```python
from build123d import *

# Parameters (mm, degrees)
SKETCH1_W           = 235
SKETCH1_H           = 120
BOSS_EXTRUDE1_DEPTH = 10
SKETCH2_R           = 15
CUT_EXTRUDE1_DEPTH  = 10
SKETCH3_R           = 2.5
CUT_EXTRUDE2_DEPTH  = 10


with BuildPart() as part:
    # Sketch1 → Boss-Extrude1 (new body)
    with BuildSketch(Plane.XY):
        Rectangle(SKETCH1_W, SKETCH1_H)
    extrude(amount=BOSS_EXTRUDE1_DEPTH)

    # Sketch2 → Cut-Extrude1 (cut)
    with BuildSketch(Plane.XY.offset(10)):
        Circle(SKETCH2_R)
    extrude(amount=-CUT_EXTRUDE1_DEPTH, mode=Mode.SUBTRACT)

    # Sketch3 → Cut-Extrude2 (cut)
    with BuildSketch(Plane.XY.offset(10)):
        with Locations((31.819805153, 31.819805153)):
            Circle(SKETCH3_R)
        with Locations((31.819805153, -31.819805153)):
            Circle(SKETCH3_R)
        with Locations((-31.819805153, -31.819805153)):
            Circle(SKETCH3_R)
        with Locations((-31.819805153, 31.819805153)):
            Circle(SKETCH3_R)
    extrude(amount=-CUT_EXTRUDE2_DEPTH, mode=Mode.SUBTRACT)


solid = part.part
```
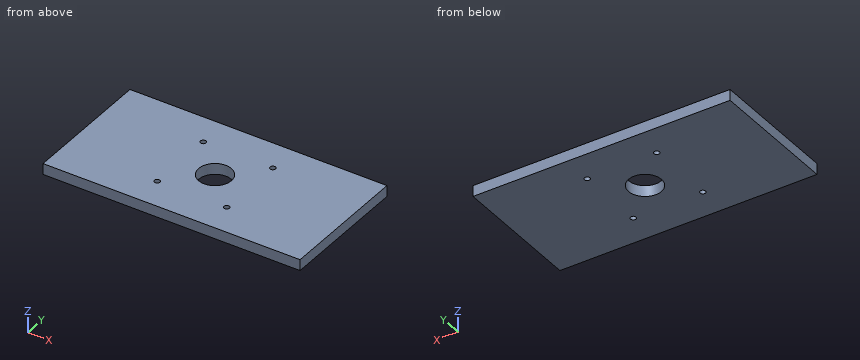
Input: part model. Units: mm. Frame: model coordinates. Give positions to 0.01 mm unless a question says otherwise; leave off trailing zeros. Loops run counter-clockwise (first coordinate to the right, second up) from the corner with the lowest first, then second, coordinate; pieces in that order, holes last.
1) Line query: L1, parallel to X at y = 0.5, z = 7.25; L2, parallel to X at y = -30, z = 0.5; L3, parallel to X at y = -2.5, z = 0.5. Output: solid intervals per line, ascending.
A:
L1: x = -117.5 to -14.99, 14.99 to 117.5
L2: x = -117.5 to -33.53, -30.11 to 30.11, 33.53 to 117.5
L3: x = -117.5 to -14.79, 14.79 to 117.5
2) Section query A-A on x = 0. Return the cut outline in (y, z).
A:
outline: (-60, 0) - (-15, 0) - (-15, 10) - (-60, 10) - close; (15, 0) - (60, 0) - (60, 10) - (15, 10) - close
3) Contact query for a flat-ended pin moving along its axis: pin 1 (8 mm diameter, centred on x = -91.5, y = -32.5, fed in from -Z). Output: stop coordinate, or through.
A:
pin 1: stops at z = 0
4) Section query B-B on y = 0. Return the cut outline in (x, z).
A:
outline: (-117.5, 0) - (-15, 0) - (-15, 10) - (-117.5, 10) - close; (15, 0) - (117.5, 0) - (117.5, 10) - (15, 10) - close
5) Section query C-C on z = 5.5. Return the cut outline in (x, y), and give its area (3 significant figures).
A:
outline: (-117.5, -60) - (117.5, -60) - (117.5, 60) - (-117.5, 60) - close; hole circle Ø5 at (-31.82, -31.82); hole circle Ø5 at (-31.82, 31.82); hole circle Ø30 at (0, 0); hole circle Ø5 at (31.82, -31.82); hole circle Ø5 at (31.82, 31.82)
area: 27,400 mm2
